Can you work these out from the model? Positions are in its coordinate system, mm. Face numbers are marked on the shaded views. Round coordinates to 2 decimals unless told otherwise and drop trailing zeros. Write each loop counter-clockwise with the first axis right and the second up, starting at its lowest first coordinate (ties: lowest second). Pieces come first, ordered by that corner, then holes.
Q1. We'd pull the mould along X, two halves only. Please class the marked faces 1, 2 and 3: +X half, -X half, draft (parallel to the pull), parting line (faces both ways), or undercut.
Q2. Please list where these lines run through material, in increasing order: line 1 along X through (y, z) = (119, 1.35); line 2 along X through (y, z) = (118.25, 0.7); line 3 along Y through (x, z) = (19.5, 0.6).
Q3. If we section it at A-A (y = 119): Please give me the cut outline in (x, z), plus the area to 3 significant figures.
Q4. If we section it at B-B (x = 31.5): Please give me the cut outline in (y, z).
Q5. If we section it at C-C (y = 135.75): Please give me the cut outline in (x, z), plus the area to 3 significant figures.
Q6. If we section it at D-D (z = 0.95): Please give me the cut outline in (x, y).
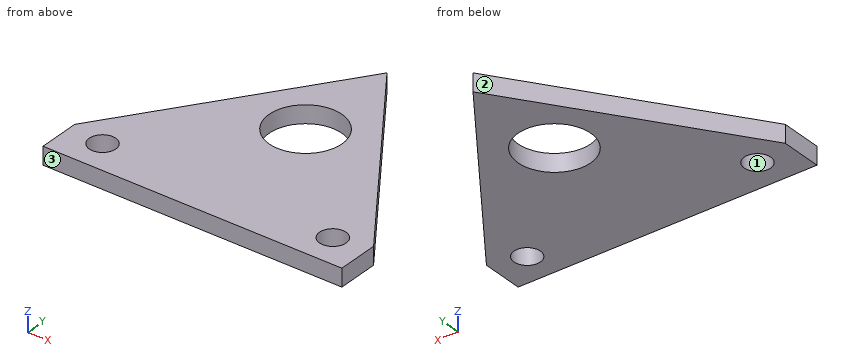
Autodesk Inventor part; units mm, degrees
ref_plane "YZ Plane" through (0, 0, 0) normal (1, 0, 0) x (0, 1, 0)
ref_plane "XZ Plane" through (0, 0, 0) normal (0, 1, 0) x (-1, 0, 0)
ref_plane "XY Plane" through (0, 0, 0) normal (0, 0, 1) x (1, 0, 0)
ref_plane "РабПлоскость1" through (0, 0, 0) normal (0, 0, 1) x (1, 0, 0)
sketch "Эскиз1" plane through (0, 0, 0) normal (0, 0, 1) x (1, 0, 0)
  line L0 (1.0452, 115.4021) -> (1.0452, 120.0556)
  line L1 (1.0452, 120.0556) -> (17.9158, 143.9758)
  line L2 (17.9158, 143.9758) -> (34.7864, 120.0556)
  line L3 (34.7864, 120.0556) -> (34.7864, 115.4021)
  line L4 (34.7864, 115.4021) -> (1.0452, 115.4021)
  circle A0 centre (5, 119) radius 1.5
  circle A1 centre (31, 119) radius 1.5
  circle A2 centre (17.9158, 132.0157) radius 4.1064
  point P0 (0, 0)
extrude "Выдавливание1" add sketch "Эскиз1" along normal blind 2
properties part number "крепеж подшипника"
A:
1. face 1: undercut
1. face 2: -X half
1. face 3: draft
2. line 1: x = 1.05 to 3.5, 6.5 to 29.5, 32.5 to 34.79
2. line 2: x = 1.05 to 3.7, 6.3 to 29.7, 32.3 to 34.79
2. line 3: y = 115.4 to 128.23, 135.8 to 141.73
3. outline: (1.05, 0) - (3.5, 0) - (3.5, 2) - (1.05, 2) - close; (6.5, 0) - (29.5, 0) - (29.5, 2) - (6.5, 2) - close; (32.5, 0) - (34.79, 0) - (34.79, 2) - (32.5, 2) - close
3. area: 55.5 mm2
4. outline: (115.4, 0) - (117.59, 0) - (117.59, 2) - (115.4, 2) - close; (120.41, 0) - (124.72, 0) - (124.72, 2) - (120.41, 2) - close
5. outline: (12.11, 0) - (16.21, 0) - (16.21, 2) - (12.11, 2) - close; (19.62, 0) - (23.72, 0) - (23.72, 2) - (19.62, 2) - close
5. area: 16.4 mm2
6. outline: (1.05, 115.4) - (34.79, 115.4) - (34.79, 120.06) - (17.92, 143.98) - (1.05, 120.06) - close; hole circle Ø3 at (5, 119); hole circle Ø8.21 at (17.92, 132.02); hole circle Ø3 at (31, 119)
